Verification items for the finished model (mm, model axes). Coordinates: 2 decimals unless noted, no trailing zeros. Order: outer loops, then holes, each group sorted by start corner. A loop starts at its lowest first (then second) coordinate and runs counter-clockwise, first axis right, second up. Notation, with made-up numbers: (83.25, 16.25) -> (106.25, 16.25) arc R4 ccw to (106.25, 21.25) -> close; hole circle Ø10 at (-32.5, 38.25). An arc over 180 degrees is marked (long way). Write each question's results on one line, items separated by ' | '. Start each with the question number.
(1) Cross-section at C-C on y = 167. Enter the section's corners in (x, z).
(2) Draft check along Z on faces 1 (the flat face through (-171, 199, -103)), 2 (the flat face through (-192, 187, 0)), 3 (the flat face through (-187, 192, -293.75)), 4 (the flat face through (-184.231, 192.122, -148.931)). Enter one of: +Z half, -Z half, draft (parallel to the pull), parting line (faces both ways), or undercut.
(3) Cross-section at D-D on z = -127.5. Enter the section's corners in (x, y).
(4) Cross-section at A-A on x = -163.5. Enter the section's corners in (y, z).
(5) Cross-section at B-B on z = -176. Enter the section's corners in (x, y), and give its area (3 significant figures).
(6) Thickness scan on probe 1 along Z at (x, y) = (-176.5, 196.5); probe 2 along Z at (x, y) = (-179, 195.5); probe 3 along Y at (x, z) = (-187.5, -198). Record the ranges inside material, lowest first. Write a range as [from, to].
(7) Go/stop test with flat-tipped pins: pin 1 (3 mm diameter, centred on x = -178, z = -202, fed in from -Y); pin 2 (6 mm diameter, centred on y = 184.5, z = -121, fed in from -X); pin 3 (12 mm diameter, centred on y = 193.5, z = -132, fed in from +X). Record where each tip stops, or that it passes through.
Autodesk Inventor part; units mm, degrees
ref_plane "YZ Plane" through (0, 0, 0) normal (1, 0, 0) x (0, 1, 0)
ref_plane "XZ Plane" through (0, 0, 0) normal (0, 1, 0) x (-1, 0, 0)
ref_plane "XY Plane" through (0, 0, 0) normal (0, 0, 1) x (1, 0, 0)
sketch "Sketch4" plane through (0, 0, 0) normal (0, 0, 1) x (1, 0, 0)
  line L0 (-193.637817, 193.637817) -> (0, 273.845227) construction
  line L1 (0, 273.845227) -> (193.637817, 193.637817) construction
  line L2 (193.637817, 193.637817) -> (273.845227, 0) construction
  line L3 (273.845227, 0) -> (193.637817, -193.637817) construction
  line L4 (193.637817, -193.637817) -> (0, -273.845227) construction
  line L5 (0, -273.845227) -> (-193.637817, -193.637817) construction
  line L6 (-193.637817, -193.637817) -> (-273.845227, 0) construction
  line L7 (-273.845227, 0) -> (-193.637817, 193.637817) construction
  line L8 (-191.341716, 191.341716) -> (0, 270.59805) construction
  line L9 (0, 270.59805) -> (191.341716, 191.341716) construction
  line L10 (191.341716, 191.341716) -> (270.59805, 0) construction
  line L11 (270.59805, 0) -> (191.341716, -191.341716) construction
  line L12 (191.341716, -191.341716) -> (0, -270.59805) construction
  line L13 (0, -270.59805) -> (-191.341716, -191.341716) construction
  line L14 (-191.341716, -191.341716) -> (-270.59805, 0) construction
  line L15 (-270.59805, 0) -> (-191.341716, 191.341716) construction
  line L16 (-189.810982, 191.975767) -> (-159.653707, 204.467319)
  line L17 (-191.975767, 189.810982) -> (-204.467319, 159.653707)
  arc A0 (-189.810982, 191.975767) -> (-191.975767, 189.810982) centre (-188.280249, 188.280249) ccw
  point P0 (0, 0)
  point P1 (0, 0)
  point P2 (0, 0)
  dimension "d16" = 506
  dimension "d22" = 3
  dimension "d23" = 32.642
  dimension "d24" = 4
contour flange "Contour Flange1" sketch "Sketch4" thickness 2 bend radius 2 width 2006 along (0, 0, -1) mid plane no both sides no wall seen from (-174.732345, 198.221543, 0) lies toward (0.3826834, -0.9238795, 0) curves L16 A0 L17
bend "Bend2"
corner "Corner2"
sketch "Sketch6" plane through (-189.810982, 191.975767, 0) normal (-0.3826834, 0.9238795, 0) x (0.9238795, 0.3826834, 0)
  circle A0 centre (16.321, 40.75) radius 5.5
  line L0 (32.642, 0) -> (0, 0)
  circle A1 centre (16.321, 1965.25) radius 5.5
  line L1 (32.642, 2006) -> (0, 2006)
  point P0 (101.896536, 0)
  point P1 (16.321, 0)
  point P2 (16.321, 0)
  point P3 (16.321, 0)
  point P4 (16.321, 0)
  point P5 (16.321, 2006)
  point P6 (16.321, 2006)
  dimension "d36" = 11
  dimension "d37" = 40.75
  dimension "d40" = 40.75
  dimension "d41" = 11
extrude "Extrusion1" cut sketch "Sketch6" against normal up to surface (2 mm away)
sketch "Sketch10" plane through (-189.810982, 191.975767, 0) normal (-0.3826834, 0.9238795, 0) x (0.9238795, 0.3826834, 0)
  line L0 (7.642, 1153) -> (32.642, 1153)
  line L1 (32.642, 1153) -> (32.642, 1103)
  line L2 (32.642, 1103) -> (7.642, 1103)
  line L3 (7.642, 1103) -> (7.642, 1153)
  line L4 (32.642, 2006) -> (0, 2006)
  line L5 (0, 0) -> (0, 2006)
  point P0 (0, 1003)
  point P1 (7.642, 1128)
  dimension "d70" = 50
  dimension "d71" = 25
  dimension "d72" = 125
extrude "Extrusion5" cut sketch "Sketch10" against normal through all
sketch "Sketch12" plane through (-191.975767, 189.810982, -2006) normal (-0.9238795, 0.3826834, 0) x (0, 0, 1)
  line L0 (853, -32.642) -> (903, -32.642)
  line L1 (903, -32.642) -> (903, -7.642)
  line L2 (903, -7.642) -> (853, -7.642)
  line L3 (853, -7.642) -> (853, -32.642)
  line L4 (2006, 0) -> (0, 0)
  point P0 (2006, -101.896536)
  point P1 (0, -32.642)
  point P2 (1003, 0)
  point P3 (878, -7.642)
  dimension "d75" = 50
  dimension "d76" = 25
  dimension "d77" = 125
extrude "Extrusion6" cut sketch "Sketch12" against normal through all
pattern_linear "Rectangular Pattern4" count 8 spacing 250 along (0, 0, 1) of "Extrusion6", "Extrusion5" first direction both ways yes
sketch "Sketch13" plane through (-189.810982, 191.975767, 0) normal (-0.3826834, 0.9238795, 0) x (0.9238795, 0.3826834, 0)
  circle A0 centre (16.321, 1003) radius 5.5
  line L0 (32.642, 903) -> (32.642, 1103)
  line L1 (32.642, 0) -> (0, 0)
  point P0 (101.896536, 0)
  point P1 (32.642, 1003)
  point P2 (16.321, 0)
  dimension "d83" = 11
extrude "Extrusion7" cut sketch "Sketch13" against normal through all
pattern_linear "Rectangular Pattern5" count 7 spacing 250 along (0, 0, 1) of "Extrusion7" first direction both ways yes
sketch "Sketch14" plane through (0, 0, 0) normal (0, 1, 0) x (-1, 0, 0)
  line L0 (-300, 0) -> (300, 0) construction
  line L1 (300, 0) -> (300, -1712.25)
  line L2 (300, -1712.25) -> (-300, -1712.25)
  line L3 (-300, -1712.25) -> (-300, 0)
  line L4 (159.653707, -2006) -> (189.810982, -2006)
  line L5 (300, -293.75) -> (-300, -293.75)
  line L6 (300, -2006) -> (-300, -2006)
  line L7 (-300, -2006) -> (-300, -1712.25)
  line L8 (300, -2006) -> (300, -1712.25)
  point P0 (0, 0)
  point P1 (0, 0)
  dimension "d89" = 600
  dimension "d90" = 1712.25
  dimension "d94" = 293.75
  dimension "d95" = 293.75
extrude "Extrusion8" cut sketch "Sketch14" along normal blind 600
equation "\"d16\" = Барабан_габарит_по_кассетам"
equation "\"d24\" = BendRadius + Thickness"
equation "\"d41\" = d36"
equation "\"d70\" = Ширина_окна_барабан"
equation "\"d75\" = Ширина_окна_барабан"
equation "\"d25\" = Thickness"
equation "\"d26\" = BendReliefWidth"
equation "\"d27\" = BendReliefDepth"
equation "\"d28\" = MinimumRemnant"
equation "\"d29\" = TransitionRadius"
equation "\"d30\" = Барабан_длина_листа"
equation "\"d31\" = BendRadius"
equation "\"d33\" = CornerReliefSize"
equation "\"d34\" = GapSize"
equation "\"d35\" = JacobiRadiusSize"
equation "\"BendRadius\" = Thickness"
equation "\"BendReliefWidth\" = Thickness"
equation "\"BendReliefDepth\" = 0.5 * Thickness"
equation "\"CornerReliefSize\" = 4 * Thickness"
equation "\"MinimumRemnant\" = 2 * Thickness"
equation "\"TransitionRadius\" = BendRadius"
equation "\"JacobiRadiusSize\" = BendRadius"
equation "\"GapSize\" = Thickness"
properties part number "ДМС 103 Полка для крышки ПВГ"
Results are:
1) outline: (-201.42, -293.75) -> (-199.26, -293.75) -> (-199.26, -153) -> (-201.42, -153) -> close; (-201.42, -103) -> (-199.26, -103) -> (-199.26, 0) -> (-201.42, 0) -> close
2) face 1: undercut | face 2: +Z half | face 3: -Z half | face 4: draft
3) outline: (-194.9, 182.75) -> (-193.05, 181.99) -> (-190.13, 189.05) arc R2 cw to (-189.05, 190.13) -> (-181.99, 193.05) -> (-182.75, 194.9) -> (-189.81, 191.98) arc R4 ccw to (-191.98, 189.81) -> close
4) outline: (200.71, -293.75) -> (202.87, -293.75) -> (202.87, -153) -> (200.71, -153) -> close; (200.71, -103) -> (202.87, -103) -> (202.87, 0) -> (200.71, 0) -> close
5) outline: (-204.47, 159.65) -> (-202.62, 158.89) -> (-190.13, 189.05) arc R2 cw to (-189.05, 190.13) -> (-158.89, 202.62) -> (-159.65, 204.47) -> (-189.81, 191.98) arc R4 ccw to (-191.98, 189.81) -> close | area: 135 mm2
6) probe 1: z = [-293.75, -258], [-248, -153], [-103, -45.75], [-35.75, 0] | probe 2: z = [-293.75, -255.33], [-250.67, -153], [-103, -43.08], [-38.42, 0] | probe 3: y = [190.77, 192.93]
7) pin 1: stops at y = 194.08 | pin 2: stops at x = -194.9 | pin 3: stops at x = -181.99
